from build123d import *

# Parameters (mm, degrees)
F0_W     = 63.5
F0_H     = 25.4
F1_DEPTH = 12.7
F2_R     = 2.1209
F3_DEPTH = 25.4
F4_R     = 2.1209
F5_DEPTH = 25.4
F6_R     = 2.1209
F7_DEPTH = 25.4


with BuildPart() as f1:
    # F0 (on Right) → F1 (new body)
    with BuildSketch(Plane.YZ):
        with Locations((0.840706, -12.7)):
            Rectangle(F0_W, F0_H)
    extrude(amount=F1_DEPTH)

    # F2 (on face) → F3 (cut)
    with BuildSketch(Plane.XY):
        with Locations((5.956479, 24.791827)):
            Circle(F2_R)
    extrude(amount=-F3_DEPTH, mode=Mode.SUBTRACT)

    # F4 (on face) → F5 (cut)
    with BuildSketch(Plane.XY):
        with Locations((6.136879, -23.729375)):
            Circle(F4_R)
    extrude(amount=-F5_DEPTH, mode=Mode.SUBTRACT)

    # F6 (on face) → F7 (cut)
    with BuildSketch(Plane.YZ.offset(12.7)):
        with Locations((0, -12.7)):
            Circle(F6_R)
    extrude(amount=-F7_DEPTH, mode=Mode.SUBTRACT)


solid = f1.part
Part model, mm, in its own coordinate system. Coordinates: 2 decimals unless noted, no trailing zeros. Write each loop counter-clockwise with the first axis right and the second up, starting at its lowest first coordinate (ties: lowest second). Pieces come first, ordered by that corner, then holes. Notation, with made-up numbers: M 85,32.25 L 104,32.25 A12 ccw 104,46.25 Z; hole C 81,44 d4. An arc over 180 degrees is marked long. Return JSON: item names as keys, results as strings.
1. Probe L1, parallel to Y at x = 4.75, z = -6.25; L2, parallel to Z at x = 4.75, y = 0; L3, parallel to Y at x = 11.75, z = -12. List the from-to ranges inside material, lowest first.
Determined:
{"L1": "-30.91 to -25.33, -22.12 to 23.05, 26.54 to 32.59", "L2": "-25.4 to -14.82, -10.58 to 0", "L3": "-30.91 to -2, 2 to 32.59"}
2. Saw through at B-B, the plane x = 6.5. Write the cut outline in (y, z), then the cut area to 3 significant figures.
Determined:
{"outline": "M -30.91,-25.4 L -25.82,-25.4 L -25.82,0 L -30.91,0 Z; M -21.64,-25.4 L 22.74,-25.4 L 22.74,0 L -21.64,0 Z; M 26.84,-25.4 L 32.59,-25.4 L 32.59,0 L 26.84,0 Z; hole C 0,-12.7 d4.24", "area": "1,390 mm²"}
3. Saw through at A-A, the plane y = 0. Write the cut outline in (x, z), then the cut area to 3 significant figures.
Determined:
{"outline": "M 0,-25.4 L 12.7,-25.4 L 12.7,-14.82 L 0,-14.82 Z; M 0,-10.58 L 12.7,-10.58 L 12.7,0 L 0,0 Z", "area": "269 mm²"}
4. Saw through at C-C, the plane z = -12.7. Write the cut outline in (x, y), then the cut area to 3 significant figures.
Determined:
{"outline": "M 0,-30.91 L 12.7,-30.91 L 12.7,-2.12 L 0,-2.12 Z; M 0,2.12 L 12.7,2.12 L 12.7,32.59 L 0,32.59 Z; hole C 5.96,24.79 d4.24; hole C 6.14,-23.73 d4.24", "area": "724 mm²"}
5. Pull direction Y, two halves, no side cores. Call faces 1 (the face through (3.838, 24.885, -12.522)), 2 (the face through (6, 0, -25.4)), 3 (the face through (6, 32.591, -13)): pulls with the +Y half, pulls with the -Y half, needs draft (parallel to the pull), parting line crosses it, or undercut.
Determined:
{"face 1": "undercut", "face 2": "needs draft", "face 3": "pulls with the +Y half"}
6. Saw through at D-D, the plane z = -8.5. Write the cut outline in (x, y), then the cut area to 3 significant figures.
Determined:
{"outline": "M 0,-30.91 L 12.7,-30.91 L 12.7,32.59 L 0,32.59 Z; hole C 5.96,24.79 d4.24; hole C 6.14,-23.73 d4.24", "area": "778 mm²"}
